Here's the drawing with two shaded views (mm, measured from the low corner). I have some questions. A direction names the side the tool comes from. Give positions to 0.01 mm unless a question says otherwise; leave off trailing zeros. Write each loop counter-clockwise with the first axis right and the second up, starting at its lowest first coordinate (ties: lowest second). Pieces come first, ordered by that corner, then holes. Notation, with made-up numbers: M 35,-24.5 L 68,-24.5 A30 ccw 68,6.5 Z; hole C 11.5,-24.75 d7. An arc over 180 degrees is marked long. Use one line per item in the form item = value.
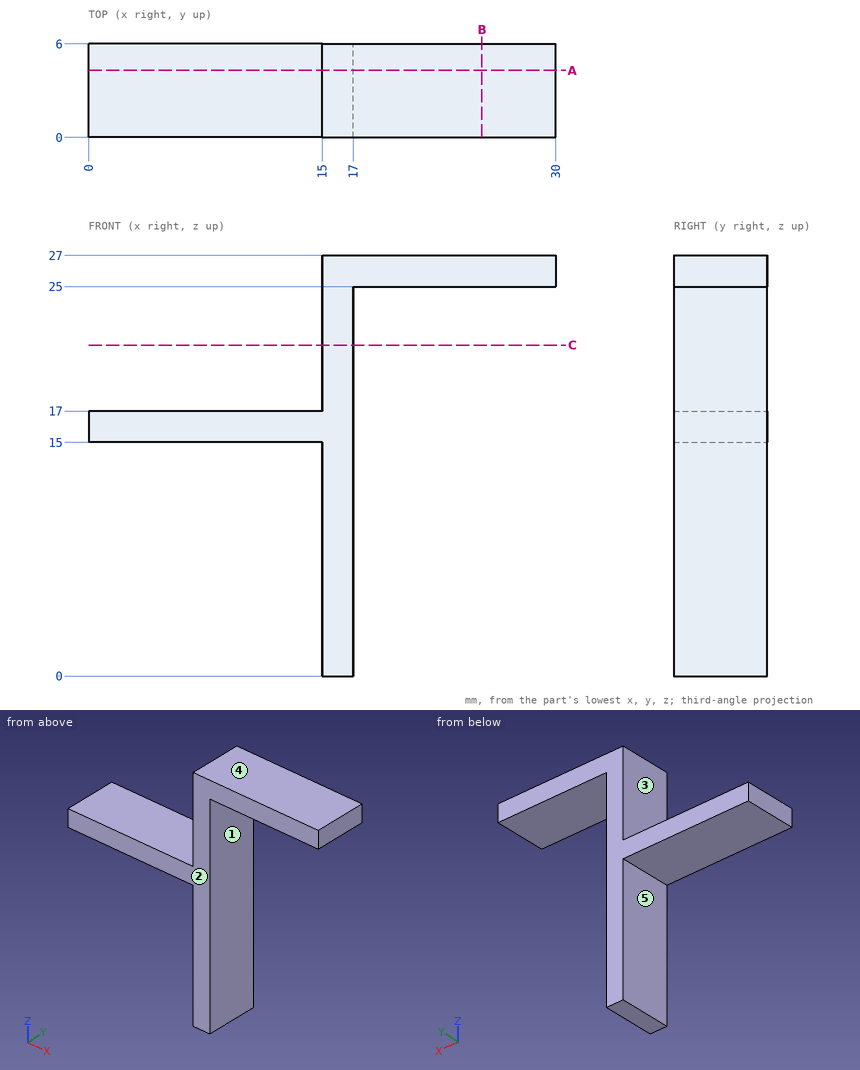
1) For pin 1 Ø1 at (y, z) = (1, 5.5) entering from -X; pin 2 Ø1 at (x, y) = (11, 3) entering from +Z; pin 3 Ø1 at (y, z) = (5, 18.5) entering from +X, each with a flat end and sliding along its axis, tell me the tip position at first contact or that it passes through.
Checked values:
pin_1 = 15
pin_2 = 17
pin_3 = 17
2) I want a section at C-C, the plane z = 21.25. Please give me the cut outline in (x, y).
Checked values:
outline = M 15,0 L 17,0 L 17,6 L 15,6 Z
3) If I drill on L1, parallel to X at y = 1.25, z = 10; L2, parallel to Z at x = 28.5, y = 3, over which ranges is the centre line in solid material (lowest first)?
Checked values:
L1 = 15 to 17
L2 = 25 to 27
4) I want a section at B-B, the plane x = 25.25. Please give me the cut outline in (y, z), plus the area to 3 significant figures.
Checked values:
outline = M 0,25 L 6,25 L 6,27 L 0,27 Z
area = 12.0 mm2
5) For the marked faces 1, 2, 3, 4 and 5, which set-ups out of +Z, -Z, +X, -X, +Y, -Y let a thin tool reach every point of the face, with its end or its side?
Checked values:
face_1 = -Z, +X, +Y, -Y
face_2 = +Z, -Z, +X, -X, -Y
face_3 = +Z, -X, +Y, -Y
face_4 = +Z, +X, -X, +Y, -Y
face_5 = -Z, -X, +Y, -Y
6) I want a section at A-A, the plane y = 4.3. Please give me the cut outline in (x, z).
Checked values:
outline = M 0,15 L 15,15 L 15,0 L 17,0 L 17,25 L 30,25 L 30,27 L 15,27 L 15,17 L 0,17 Z
